Part model, mm, in its own coordinate system. Coordinates: 2 decimals unless noted, no trailing zeros. Order: outer loops, then holes, each group sorted by start corner. A loop starts at its lowest first (then second) coordinate and runs counter-clockwise, first axis right, second up. Notation, with made-up numbers: (78.25, -38.75) - (107.25, -38.75) arc R13 cw to (107.25, -22.75) - close; hole circle Ø3 at (-37.75, 33). An arc over 180 degrees is marked (long way). Use a Markdown table: item, result. Add a question column.
1) Wall check: L1, parallel to X at y = -16.3, z = 0.5; L2, parallel to Y at x = -4, z = 1.5 (3 decimals); L3, parallel to Y at x = 15, z = 0.65. Give the ranges that are in metal, low to high. Write a range as [from, to].
2) Saw through at B-B on y = -16.3. List the corners of the cut face in (x, z), then the cut area to 3 significant figures.
3) Saw through at A-A on x = -15. List the corners of the cut face in (y, z), then the cut area to 3 significant figures.
4) Two-plate mould, pull along Y, no slides. Class faces 1 (the face through (0, 0, 0)), 2 (the face through (-14.446, -17.365, 0.813)), 3 (the face through (0, -21.8, 1)): +Y half, -Y half, draft (parallel to the pull), parting line (faces both ways), or undercut.
```python
from build123d import *

# Parameters (mm, degrees)
SKETCH1_W               = 33.5
SKETCH1_H               = 43.6
BOSS_EXTRUDE1_DEPTH     = 1.65
BOSS_EXTRUDE2_START     = -3.05
SKETCH2_W               = 0.65
SKETCH2_H               = 0.65
BOSS_EXTRUDE2_DEPTH     = 11.55
CUT_EXTRUDE1_START      = -4.05
SKETCH2_2_W             = 0.65
SKETCH2_2_H             = 0.65
CUT_EXTRUDE1_DEPTH      = 13.55
LPATTERN1_COUNT         = 4
LPATTERN1_PITCH         = 2.54
MIRROR1_START           = -4.05
MIRROR1_COPY_1_SKETCH_W = 0.65
MIRROR1_COPY_1_SKETCH_H = 0.65
MIRROR1_COPY_1_DEPTH    = 13.55
MIRROR1_COPY_2_SKETCH_W = 0.65
MIRROR1_COPY_2_SKETCH_H = 0.65
MIRROR1_COPY_2_DEPTH    = 13.55
MIRROR1_COPY_3_SKETCH_W = 0.65
MIRROR1_COPY_3_SKETCH_H = 0.65
MIRROR1_COPY_3_DEPTH    = 13.55
MIRROR1_COPY_4_SKETCH_W = 0.65
MIRROR1_COPY_4_SKETCH_H = 0.65
MIRROR1_COPY_4_DEPTH    = 13.55
SKETCH3_R               = 1.2
CUT_EXTRUDE2_DEPTH      = 2.65


with BuildPart() as part:
    # Sketch1 → Boss-Extrude1 (new body)
    with BuildSketch(Plane.XY):
        Rectangle(SKETCH1_W, SKETCH1_H)
    extrude(amount=BOSS_EXTRUDE1_DEPTH)

    # Sketch2 → Boss-Extrude2 (add)
    with BuildSketch(Plane(origin=(0, 0, 0), x_dir=(-1, 0, 0), z_dir=(0, 0, -1)).offset(BOSS_EXTRUDE2_START)):
        with Locations((-1.27, -19.55)):
            Rectangle(SKETCH2_W, SKETCH2_H)
    boss_extrude2 = extrude(amount=BOSS_EXTRUDE2_DEPTH)

    # Sketch2<2> → Cut-Extrude1 (cut)
    with BuildSketch(Plane(origin=(0, 0, 0), x_dir=(-1, 0, 0), z_dir=(0, 0, -1)).offset(CUT_EXTRUDE1_START)):
        with Locations((-1.27, -19.55)):
            Rectangle(SKETCH2_2_W, SKETCH2_2_H)
    cut_extrude1 = extrude(amount=CUT_EXTRUDE1_DEPTH, mode=Mode.SUBTRACT)

    # LPattern1: Cut-Extrude1 ×4
    with Locations(*[(i * LPATTERN1_PITCH, 0, 0) for i in range(1, LPATTERN1_COUNT)]):
        add(cut_extrude1, mode=Mode.SUBTRACT)

    # Mirror1: Boss-Extrude2 across plane
    add(boss_extrude2.mirror(Plane(origin=(0, 0, 0), x_dir=(0, 0, 1), z_dir=(1, 0, 0))))

    # Mirror1 copy 1 sketch → Mirror1 copy 1 (cut)
    with BuildSketch(Plane(origin=(-2.54, 0, 0), x_dir=(1, 0, 0), z_dir=(0, 0, -1)).offset(MIRROR1_START)):
        with Locations((-1.27, 19.55)):
            Rectangle(MIRROR1_COPY_1_SKETCH_W, MIRROR1_COPY_1_SKETCH_H)
    extrude(amount=MIRROR1_COPY_1_DEPTH, mode=Mode.SUBTRACT)

    # Mirror1 copy 2 sketch → Mirror1 copy 2 (cut)
    with BuildSketch(Plane(origin=(-5.08, 0, 0), x_dir=(1, 0, 0), z_dir=(0, 0, -1)).offset(MIRROR1_START)):
        with Locations((-1.27, 19.55)):
            Rectangle(MIRROR1_COPY_2_SKETCH_W, MIRROR1_COPY_2_SKETCH_H)
    extrude(amount=MIRROR1_COPY_2_DEPTH, mode=Mode.SUBTRACT)

    # Mirror1 copy 3 sketch → Mirror1 copy 3 (cut)
    with BuildSketch(Plane(origin=(-7.62, 0, 0), x_dir=(1, 0, 0), z_dir=(0, 0, -1)).offset(MIRROR1_START)):
        with Locations((-1.27, 19.55)):
            Rectangle(MIRROR1_COPY_3_SKETCH_W, MIRROR1_COPY_3_SKETCH_H)
    extrude(amount=MIRROR1_COPY_3_DEPTH, mode=Mode.SUBTRACT)

    # Mirror1 copy 4 sketch → Mirror1 copy 4 (cut)
    with BuildSketch(Plane(origin=(0, 0, 0), x_dir=(1, 0, 0), z_dir=(0, 0, -1)).offset(MIRROR1_START)):
        with Locations((-1.27, 19.55)):
            Rectangle(MIRROR1_COPY_4_SKETCH_W, MIRROR1_COPY_4_SKETCH_H)
    extrude(amount=MIRROR1_COPY_4_DEPTH, mode=Mode.SUBTRACT)

    # Sketch3 → Cut-Extrude2 (cut, through all)
    with BuildSketch(Plane.XY):
        with Locations((-15, -16.3)):
            Circle(SKETCH3_R)
        with Locations((15, -16.3)):
            Circle(SKETCH3_R)
    extrude(amount=CUT_EXTRUDE2_DEPTH, mode=Mode.SUBTRACT)


solid = part.part
```
Results are:
| question | item | result |
|---|---|---|
| 1 | L1 | [-16.75, -16.2], [-13.8, 13.8], [16.2, 16.75] |
| 1 | L2 | [-21.8, -19.875], [-19.225, 21.8] |
| 1 | L3 | [-21.8, -17.5], [-15.1, 21.8] |
| 2 | outline | (-16.75, 0) - (-16.2, 0) - (-16.2, 1.65) - (-16.75, 1.65) - close; (-13.8, 0) - (13.8, 0) - (13.8, 1.65) - (-13.8, 1.65) - close; (16.2, 0) - (16.75, 0) - (16.75, 1.65) - (16.2, 1.65) - close |
| 2 | area | 47.4 mm2 |
| 3 | outline | (-21.8, 0) - (-17.5, 0) - (-17.5, 1.65) - (-21.8, 1.65) - close; (-15.1, 0) - (21.8, 0) - (21.8, 1.65) - (-15.1, 1.65) - close |
| 3 | area | 68.0 mm2 |
| 4 | face 1 | draft |
| 4 | face 2 | undercut |
| 4 | face 3 | -Y half |
